Check sheet for the modelled part. Datum: model origin and axes. Units: mm. A direction names the side the tool comes from. Coordinates: 2 decimals unless noted, no trailing zeros. Loops run counter-clockwise (first coordinate to the right, second up) from the corner with the lowest first, then second, coordinate; pieces in that order, holes last. Notation, with made-up numbers: (25, 86) - (30, 86) arc R36 ccw to (30, 122) - close; hole circle Ø2 at (9.5, 61.5). An arc over 180 degrees is marked (long way). Use a Markdown table: item, result. Add a question column.
1) Sectioned sample at D-D, the plane x = -25. Enter the section's corners in (y, z), then the cut area to 3 significant figures.
2) Sectioned sample at A-A, the plane x = 6. Enter the section's corners in (y, z), then the cut area to 3 significant figures.
3) Thickness scan on line 1 (Y direction, x = 7.5, z = 16); line 2 (X direction, y = 27.25, z = 1); line 3 (Z direction, x = 22, y = 2.75). Record the ranges inside material, lowest first.
4) Go/stop test with flat-tipped pins: P1, Ø3.5, axis at y = 22, z = -22, coming from the +X side; P2, Ø3.5, axis at x = -21.5, y = 22, coming from the +Z side; P3, Ø17.5, axis at x = 7, z = 5.5, coming from the +Y side. Record where each tip stops, or that it passes through.
5) Tool access check on faces 1 (the cylindrical face through (7.94, 29.1, -14.86)), 2 (the flat face through (17, 23, -24)), 3 (the flat face through (-23, 23, 21)). Record the directions out of +Z, -Z, +X, -X, +Y, -Y that give a thin tool (end or side, any length) a straight path to the whole face; none if there is none.
6) Sectioned sample at B-B, the plane y = 3.5. Enter the section's corners in (x, z).
7) Sectioned sample at C-C, the plane z = 22. Enter the section's corners in (x, y).
Autodesk Inventor part; units mm, degrees
ref_plane "YZ Plane" through (0, 0, 0) normal (1, 0, 0) x (0, 1, 0)
ref_plane "XZ Plane" through (0, 0, 0) normal (0, 1, 0) x (-1, 0, 0)
ref_plane "XY Plane" through (0, 0, 0) normal (0, 0, 1) x (1, 0, 0)
sketch "Schizzo11" plane through (0, 0, 0) normal (0, 1, 0) x (-1, 0, 0)
  line L0 (29, -29) -> (-29, -29)
  line L1 (-29, -29) -> (-29, 9)
  line L2 (-19, 29) -> (29, 29)
  line L3 (29, 29) -> (29, -29)
  line L4 (29, -29) -> (-29, 29) construction
  line L5 (-29, -29) -> (29, 29) construction
  line L6 (29, -29) -> (29, 21)
  line L7 (29, 21) -> (16, 21)
  line L8 (11, 16) -> (11, 1)
  line L9 (29, -29) -> (-17, -29)
  line L10 (-17, -29) -> (-17, -19)
  line L11 (-12, -14) -> (-4, -14)
  arc A0 (-4, -14) -> (11, 1) centre (-4, 1) ccw
  arc A1 (16, 21) -> (11, 16) centre (16, 16) ccw
  arc A2 (-12, -14) -> (-17, -19) centre (-12, -19) ccw
  line L12 (-19, 29) -> (-29, 9)
  point P0 (0, 0)
  point P1 (11, 21)
  point P2 (11, -14)
  point P3 (-17, -14)
  dimension "d28" = 58
  dimension "d29" = 58
  dimension "d30" = 50
  dimension "d31" = 18
  dimension "d32" = 35
  dimension "d33" = 46
  dimension "d34" = 15
  dimension "d35" = 15
  dimension "d36" = 5
  dimension "d37" = 5
  dimension "d38" = 10
  dimension "d39" = 20
extrude "Estrusione6" add sketch "Schizzo11" along normal blind 30 contours L0 L10 A2 L11 A0 L8 A1 L7 L3
extrude "Estrusione7" add sketch "Schizzo11" along normal blind 20 contours L0 L1 L12 L2 L3 L7 A1 L8 A0 L11 A2 L10
fillet "Raccordo3" radius 3 7 edges at (8, 30, -14) (15.5355, 30, -15.4645) (17, 30, -24) (-11, 30, 8.5) (-12.4645, 30, 19.5355) (-22.5, 30, 21) (-6.6066, 30, -9.6066)
fillet "Raccordo4" radius 5 1 edges at (-29, 15, -29)
properties part number "primo esercizio"
Solved:
| question | item | result |
|---|---|---|
| 1 | outline | (0, -28.9) - (30, -28.9) - (30, 18) arc R3 ccw to (27, 21) - (20, 21) - (20, 29) - (0, 29) - close |
| 1 | area | 1,660 mm2 |
| 2 | outline | (0, -29) - (30, -29) - (30, -17) arc R3 ccw to (27, -14) - (20, -14) - (20, 29) - (0, 29) - close |
| 2 | area | 1,310 mm2 |
| 3 | line 1 | y = 0 to 20 |
| 3 | line 2 | x = -29 to -11.01 |
| 3 | line 3 | z = -29 to 23 |
| 4 | P1 | stops at x = 17 |
| 4 | P2 | stops at z = 21 |
| 4 | P3 | stops at y = 20 |
| 5 | face 1 | +Z, +X, +Y |
| 5 | face 2 | +Z, -Z, +X, +Y |
| 5 | face 3 | +Z, +X, -X, +Y |
| 6 | outline | (-29, -24) arc R5 ccw to (-24, -29) - (29, -29) - (29, 9) - (19, 29) - (-29, 29) - close |
| 7 | outline | (-29, 0) - (22.5, 0) - (22.5, 20) - (-29, 20) - close |
